```python
from build123d import *

# Parameters (mm, degrees)
F0_W     = 127
F0_H     = 127
F1_DEPTH = 12.7
F2_W     = 127
F2_H     = 127
F3_DEPTH = 25.4


with BuildPart() as f1:
    # F0 (on Top) → F1 (new body)
    with BuildSketch(Plane.XY):
        with Locations((-5.2748060389, -3.7782490253)):
            Rectangle(F0_W, F0_H)
    extrude(amount=F1_DEPTH)

    # F2 (on face) → F3 (cut)
    with BuildSketch(Plane.XY.offset(12.7)):
        with Locations((-5.2748060389, -3.7782490253)):
            Rectangle(F2_W, F2_H)
        with BuildLine():
            ThreePointArc((-45.0568873794, 18.5549733723), (-21.680808978, 40.5123780124), (5.5957227014, 23.6434871331))
            ThreePointArc((5.5957227014, 23.6434871331), (20.7619644282, 23.9522780163), (35.3910028934, 27.9649421573))
            ThreePointArc((35.3910028934, 27.9649421573), (38.3541893018, 22.3998611891), (36.5282259881, 16.3652561605))
            ThreePointArc((36.5282259881, 16.3652561605), (21.5049263239, 17.0007372687), (6.9639624681, 13.1714110634))
            ThreePointArc((6.9639624681, 13.1714110634), (10.555668828, 1.3136130229), (12.6937493314, -10.8903347278))
            ThreePointArc((12.6937493314, -10.8903347278), (6.4730682144, -13.9075075331), (0, -16.3364153508))
            ThreePointArc((0, -16.3364153508), (-3.1058492811, -17.2664709372), (-6.2491420152, -18.060834795))
            Line((-6.2491420152, -18.060834795), (-4.7052248427, -24.6445921262))
            Line((-4.7052248427, -24.6445921262), (-0.2844387127, -23.6079002679))
            Line((-0.2844387127, -23.6079002679), (0.160669737, -25.505985263))
            Line((0.160669737, -25.505985263), (-6.4033689389, -27.0452783327))
            Line((-6.4033689389, -27.0452783327), (-8.4020764283, -18.5221494234))
            ThreePointArc((-8.4020764283, -18.5221494234), (-12.6823960096, -19.2448601378), (-16.9974779801, -19.7176328979))
            ThreePointArc((-16.9974779801, -19.7176328979), (-20.2884334166, -19.9086672669), (-23.5846133504, -19.9542705577))
            Line((-23.5846133504, -19.9542705577), (-22.1019901652, -26.276650695))
            Line((-22.1019901652, -26.276650695), (-17.6166596284, -25.2248229177))
            Line((-17.6166596284, -25.2248229177), (-17.1715511787, -27.1229079127))
            Line((-17.1715511787, -27.1229079127), (-23.7623452954, -28.6684752393))
            Line((-23.7623452954, -28.6684752393), (-25.8180133273, -19.9024483329))
            ThreePointArc((-25.8180133273, -19.9024483329), (-31.5468119996, -19.4625349649), (-37.2248290455, -18.5834556595))
            ThreePointArc((-37.2248290455, -18.5834556595), (-38.4809946553, -15.7990470828), (-39.6320844368, -12.9695815014))
            Line((-39.6320844368, -12.9695815014), (-48.9112883806, -17.4878127873))
            Line((-48.9112883806, -17.4878127873), (-58.4690012038, 11.1827589571))
            add(Edge.make_bspline(
                [(-58.4690012038, 11.1827589571), (-58.2366652986, 17.2623036133), (-57.6099015071, 28.8951190176), (-49.4002085789, 21.9963852094), (-45.0568873794, 18.5549733723)],
                knots=[0, 0, 0, 0, 0.5142248233, 1, 1, 1, 1], degree=3))
        make_face(mode=Mode.SUBTRACT)
    extrude(amount=-F3_DEPTH, mode=Mode.SUBTRACT)


solid = f1.part
```
The model under review builds one solid part; all positions refer to its coordinate system, in mm. A direction names the side the tool comes from. Give positions to 0.01 mm unless a question says otherwise; leave off trailing zeros. Loops run counter-clockwise (first coordinate to the right, second up) from the corner with the lowest first, then second, coordinate; pieces in that order, holes last. Notation, with made-up numbers: (2.25, 61.25) - (20.25, 61.25) arc R33 cw to (20.25, 96.25) - close; hole circle Ø7 at (4, 25.5). An arc over 180 degrees is marked (long way). Answer as a JSON object with one key per item and string values.
Q1. Insertion check: pin 1 (1 mm diameter, centred on y = 14.5, z = 7.5, fed in from -X); pin 2 (6 mm diameter, centred on x = -5, z = 8.5, fed in from +Y); pin 3 (3 mm diameter, centred on y = -0.5, z = 5.5, fed in from -X). Each pin has a flat end and moves straight along its axis. Give the tip position at first contact, or say it passes through.
Worked out:
{"pin 1": "stops at x = -58.35", "pin 2": "stops at y = 38.22", "pin 3": "stops at x = -55.07"}
Q2. Mouldability with a two-part tool opening along X and no side actions: class faces 1 (the flat face through (-21, 6, 0)), 2 (the cylindrical face through (10.515, 1.482, 6.439)), 3 (the cylindrical face through (-38.464, -15.838, 6.439)), 4 (the cylindrical face through (21.715, 17.023, 6.439)) as +X half, -X half, draft (parallel to the pull), parting line (faces both ways), or undercut.
Worked out:
{"face 1": "draft", "face 2": "+X half", "face 3": "undercut", "face 4": "undercut"}
Q3. Add section A-A on x = 8. State the section outline as (y, z) points, plus the area to 3 significant figures.
Worked out:
{"outline": "(-13.23, 0) - (10.24, 0) - (10.24, 12.7) - (-13.23, 12.7) - close; (13.6, 0) - (23.44, 0) - (23.44, 12.7) - (13.6, 12.7) - close", "area": "423 mm^2"}
Q4. To check wall thickness, follow line 1 along Y through (x, z) = (-26, 6.5); line 2 along Y through (x, z) = (-37.5, 1.5); line 3 along X through (y, z) = (-8.5, 9.5). State the ranges of each line that lie inside material, in increasing order.
Worked out:
{"line 1": "y = -19.9 to 39.71", "line 2": "y = -18 to 33.11", "line 3": "x = -51.91 to 12.39"}
Q5. Add section D-D on y = 31.5. State the section outline as (x, z) points, plus the area to 3 significant figures.
Worked out:
{"outline": "(-39.01, 0) - (0.92, 0) - (0.92, 12.7) - (-39.01, 12.7) - close", "area": "507 mm^2"}
Q6. For faces 5 (the cylindrical face through (3.6, -15.07, 6.44)), 6 (the flat face through (-44.21, -15.2, 6.44)), 7 (the flat face through (-24.776, -24.347, 6.439)), 8 (the flat face through (-19.891, -25.758, 6.439)), list the 3-axis set-ups (+Z, -Z, +X, -X, +Y, -Y) from which the entire face can be reached by the end or side of a thin tool; tool diameter is ignored.
Worked out:
{"face 5": "+Z, -Z, +X", "face 6": "+Z, -Z, -Y", "face 7": "+Z, -Z, -X, -Y", "face 8": "+Z, -Z"}
Q7. Add section B-B on y = -21. State the section outline as (x, z) points.
Worked out:
{"outline": "(-25.56, 0) - (-23.34, 0) - (-23.34, 12.7) - (-25.56, 12.7) - close; (-7.82, 0) - (-5.56, 0) - (-5.56, 12.7) - (-7.82, 12.7) - close"}
Q8. Add section C-C on x = 26. State the section outline as (y, z) points, plus the area to 3 significant figures.
Worked out:
{"outline": "(17.28, 0) - (24.95, 0) - (24.95, 12.7) - (17.28, 12.7) - close", "area": "97.3 mm^2"}
